Design review of the part shown in the three views and the two pictorial views. Dimensions are in mm from the part's minimum x, y and z. A direction names the side the tool comes from. Round coordinates to 2 decimals unless told otherwise and drop trailing zeros. Order: outer loops, then holes, each group sorted by start corner. A loop starts at its lowest first (then second) coordinate and runs counter-clockwise, first axis right, second up.
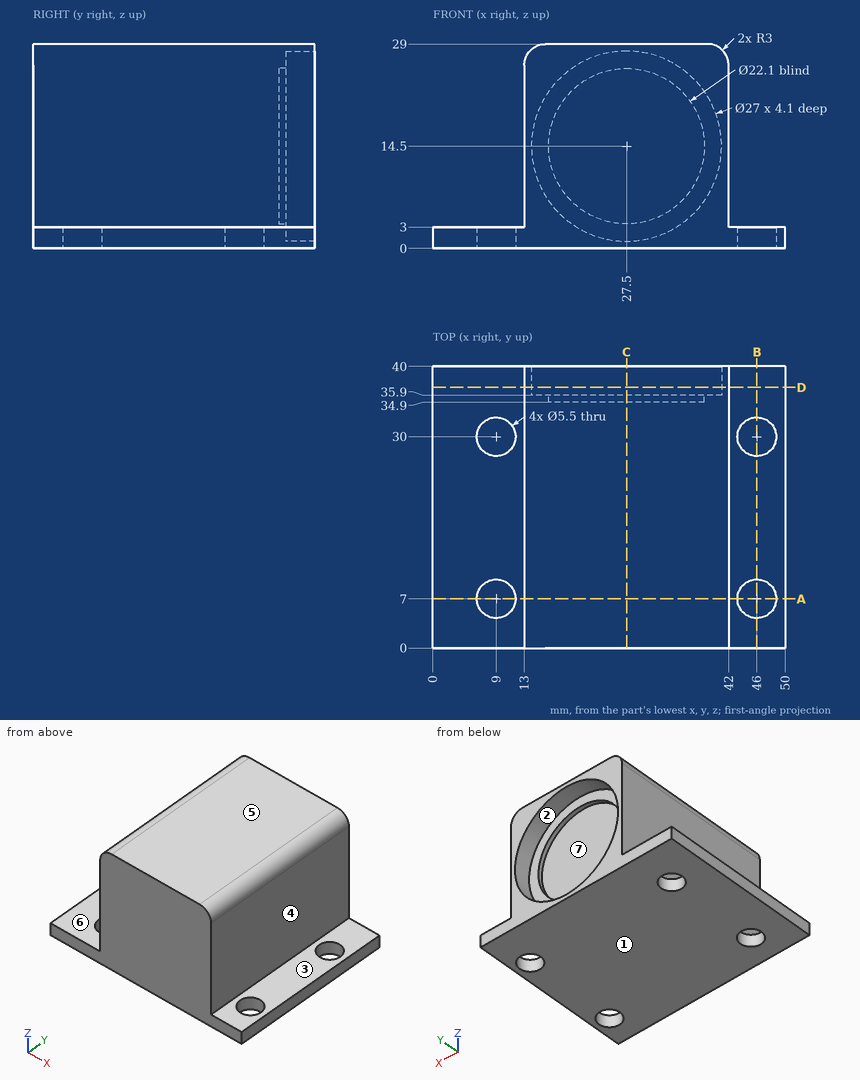
1) Take a section at A-A on y = 7. Give the boundary of the cut face in (x, z).
Results:
outline: (0, 0) - (6.25, 0) - (6.25, 3) - (0, 3) - close; (11.75, 0) - (43.25, 0) - (43.25, 3) - (42, 3) - (42, 26) arc R3 ccw to (39, 29) - (16, 29) arc R3 ccw to (13, 26) - (13, 3) - (11.75, 3) - close; (48.75, 0) - (50, 0) - (50, 3) - (48.75, 3) - close
2) Take a section at C-C on x = 27.5. Give the boundary of the cut face in (y, z).
Results:
outline: (0, 0) - (40, 0) - (40, 1) - (35.9, 1) - (35.9, 3.45) - (34.9, 3.45) - (34.9, 25.55) - (35.9, 25.55) - (35.9, 28) - (40, 28) - (40, 29) - (0, 29) - close
3) Take a section at D-D on y = 37. Give the boundary of the cut face in (x, z).
Results:
outline: (0, 0) - (50, 0) - (50, 3) - (42, 3) - (42, 26) arc R3 ccw to (39, 29) - (16, 29) arc R3 ccw to (13, 26) - (13, 3) - (0, 3) - close; hole circle Ø27 at (27.5, 14.5)
4) For the marked faces 4, 5, 6 and 7, list the 3-axis set-ups (+Z, -Z, +X, -X, +Y, -Y) from which the entire face can be reached by the end or side of a thin tool; tool diameter is ignored.
Results:
face 4: +Z, +X, +Y, -Y
face 5: +Z, +X, -X, +Y, -Y
face 6: +Z, -X, +Y, -Y
face 7: +Y
5) To check wall thickness, follow line 1 along Y through (x, z) = (9, 1.1); line 2 along X through (y, z) = (38.75, 14.5); line 3 along X through (y, z) = (11.5, 9.75). State the ranges of each line that lie inside material, in increasing order.
Results:
line 1: y = 0 to 4.25, 9.75 to 27.25, 32.75 to 40
line 2: x = 13 to 14, 41 to 42
line 3: x = 13 to 42
6) Clearance check with flat-ended pins moving along their axes: P1, Ø1.5, axis at y = 27, z = 21, coming from the +X side; P2, Ø7, axis at y = 27.5, z = 20, coming from the -X side; P3, Ø10, axis at x = 10, y = 31, coming from the +Z side. State where each tip first meets the part, or that it passes through.
Results:
P1: stops at x = 42
P2: stops at x = 13
P3: stops at z = 28.83
7) Take a section at B-B on x = 46. Give the boundary of the cut face in (y, z), plus the area to 3 significant figures.
Results:
outline: (0, 0) - (4.25, 0) - (4.25, 3) - (0, 3) - close; (9.75, 0) - (27.25, 0) - (27.25, 3) - (9.75, 3) - close; (32.75, 0) - (40, 0) - (40, 3) - (32.75, 3) - close
area: 87.0 mm2
8) The part is to be moulded in two halves that separate along Z. For the marked faces 1, 2 and 3, say which applies: released by +Z, released by -Z, zero draft, split by the parting line, or undercut.
Results:
face 1: released by -Z
face 2: undercut
face 3: released by +Z
